from build123d import *

# Parameters (mm, degrees)
F0_R     = 10
F1_DEPTH = 4
F2_R     = 8
F3_DEPTH = 25
F4_R     = 9
F5_DEPTH = 3.5


with BuildPart() as f1:
    # F0 (on Top) → F1 (new body)
    with BuildSketch(Plane.XY):
        Circle(F0_R)
    extrude(amount=F1_DEPTH)

    # F2 (on face) → F3 (cut)
    with BuildSketch(Plane.XY.offset(4)):
        Circle(F2_R)
    extrude(amount=-F3_DEPTH, mode=Mode.SUBTRACT)

    # F4 (on face) → F5 (cut)
    with BuildSketch(Plane(origin=(0, 0, 0), x_dir=(1, 0, 0), z_dir=(0, 0, -1))):
        Circle(F4_R)
    extrude(amount=-F5_DEPTH, mode=Mode.SUBTRACT)


solid = f1.part
Check sheet for the modelled part. Datum: model origin and axes. Units: mm. Coordinates: 2 decimals unless noted, no trailing zeros. Write each loop counter-clockwise with the first axis right and the second up, starting at its lowest first coordinate (ties: lowest second). Pieces come first, ordered by that corner, then holes. Notation, with made-up numbers: M 25.5,46 L 78.5,46 A10 ccw 78.5,65 Z; hole C -33.75,49 d10. An arc over 180 degrees is marked long. Answer as CSV lines item,"result".
Q1. Cross-section at A-A (x = 0). Record the boundary of the cut face in (y, z).
Check result:
outline,"M -10,0 L -9,0 L -9,3.5 L -8,3.5 L -8,4 L -10,4 Z; M 8,3.5 L 9,3.5 L 9,0 L 10,0 L 10,4 L 8,4 Z"
Q2. Material ranges on probe 1 along Y at (x, z) = (0, 0.8); probe 2 along Y at (x, z) = (0, 3.85); probe 3 along X at (y, z) = (-7.75, 2.9), recorded low to high. Write a range as from..to.
Check result:
probe 1,"-10..-9, 9..10"
probe 2,"-10..-8, 8..10"
probe 3,"-6.32..-4.58, 4.58..6.32"
Q3. Mould release check, pull along Y, two halves, no side actions. Record for faces 1 (the face through (-9, 2, 0)), 2 (the face through (-1.172, -8.923, 1.726)), 3 (the face through (-2.17, -9.76, 1.97)): released by +Y, released by -Y, zero draft, split by the parting line, or undercut.
Check result:
face 1,"zero draft"
face 2,"undercut"
face 3,"split by the parting line"
Q4. Cross-section at C-C (z = 2.75). Record the boundary of the cut face in (x, y).
Check result:
outline,"C 0,0 d20; hole C 0,0 d18"
Q5. Go/stop test with flat-tipped pins: pin 1 (1 mm diameter, centred on x = -6.5, z = 3, fed in from -Y); pin 2 (1 mm diameter, centred on y = 2, z = 1, fed in from -X); pin 3 (2 mm diameter, centred on y = -4.5, z = 2, fed in from -X). Record where each tip stops, or that it passes through.
Check result:
pin 1,"y = -8"
pin 2,"x = -9.89"
pin 3,"x = -9.37"
